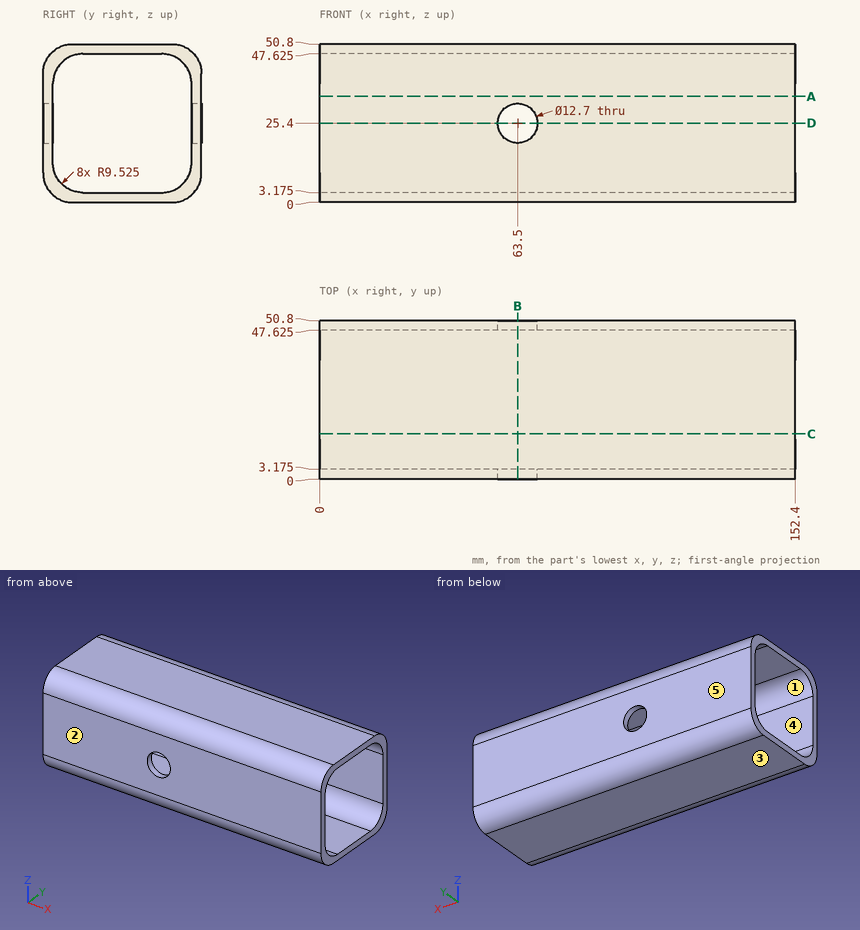
Check sheet for the drawn part. Datum: minimum x, y, z corner. Units: mm. A direction names the side the tool comes from. Round coordinates to 2 decimals unless told otherwise and drop trailing zeros. Loops run counter-clockwise (first coordinate to the right, second up) from the corner with the lowest first, then second, coordinate; pieces in that order, holes last. Notation, with made-up numbers: (0, 17) -> (12, 17) arc R34 cw to (12, 48) -> close; hole circle Ø4 at (-12.75, 2). An arc over 180 degrees is marked (long way). Put each result on its own line as item: value. Start each with the question number.
1. Section check B-B (x = 63.5). Enter the section's corners in (y, z) (3 decimals), plus the area to 3 significant figures.
2. Gauge pin test, flat ends, axial feed: pin 1 (20.5 mm diameter, centred on x = 54, y = 24, fed in from -Z); pin 2 (1 mm diameter, centred on x = 26.5, z = 8.5, fed in from +Y); pin 3 (2 mm diameter, centred on x = 79.5, z = 5.5, fed in from -Y); pin 4 (5 mm diameter, centred on x = 28, y = 6, fed in from -Z). Record the tip position at first contact, or that the pin passes through.
3. Section check D-D (z = 25.4). Enter the section's corners in (x, y) (3 decimals).
4. Section check A-A (z = 34). Enter the section's corners in (x, y) (3 decimals), plus the area to 3 significant figures.
5. Access from +Z, -Z, +X, -X, +Y, -Y to the whole of each face (thin tool, end or side, straight path). Record for the marked faces 1 and 2.
6. Draft check along Z on the marked faces 3, 4 and 5. Enter one of: +Z half, -Z half, draft (parallel to the pull), parting line (faces both ways), or undercut.
7. Scan lines: probe 1 along X at (y, z) = (1, 25); probe 2 along Y at (x, z) = (12.5, 28) (3 decimals). Record each from-to range of solid material in increasing order.
Findings:
1. outline: (0, 9.525) arc R9.525 ccw to (9.525, 0) -> (41.275, 0) arc R9.525 ccw to (50.8, 9.525) -> (50.8, 19.05) -> (47.625, 19.05) -> (47.625, 12.7) arc R9.525 cw to (38.1, 3.175) -> (12.7, 3.175) arc R9.525 cw to (3.175, 12.7) -> (3.175, 19.05) -> (0, 19.05) -> close; (0, 31.75) -> (3.175, 31.75) -> (3.175, 38.1) arc R9.525 cw to (12.7, 47.625) -> (38.1, 47.625) arc R9.525 cw to (47.625, 38.1) -> (47.625, 31.75) -> (50.8, 31.75) -> (50.8, 41.275) arc R9.525 ccw to (41.275, 50.8) -> (9.525, 50.8) arc R9.525 ccw to (0, 41.275) -> close
1. area: 524 mm^2
2. pin 1: stops at z = 0
2. pin 2: stops at y = 50.79
2. pin 3: stops at y = 0.49
2. pin 4: stops at z = 0.06
3. outline: (0, 0) -> (57.15, 0) -> (57.15, 3.175) -> (0, 3.175) -> close; (0, 47.625) -> (57.15, 47.625) -> (57.15, 50.8) -> (0, 50.8) -> close; (69.85, 0) -> (152.4, 0) -> (152.4, 3.175) -> (69.85, 3.175) -> close; (69.85, 47.625) -> (152.4, 47.625) -> (152.4, 50.8) -> (69.85, 50.8) -> close
4. outline: (0, 0) -> (152.4, 0) -> (152.4, 3.175) -> (0, 3.175) -> close; (0, 47.625) -> (152.4, 47.625) -> (152.4, 50.8) -> (0, 50.8) -> close
4. area: 968 mm^2
5. face 1: +X, -X
5. face 2: +Z, -Z, +X, -X, -Y
6. face 3: -Z half
6. face 4: undercut
6. face 5: draft
7. probe 1: x = 0 to 57.16, 69.84 to 152.4
7. probe 2: y = 0 to 3.175, 47.625 to 50.8
